Verification items for the finished model (mm, model axes). Face numbers are marked on the shaded views. A direction names the side the tool comes from. Coordinates: 2 decimals unless noted, no trailing zeros. Order: outer loops, then holes, each group sorted by start corner. A loop starts at its lowest first (then second) coordinate and runs counter-clockwise, first axis right, second up. Notation, with made-up numbers: M 25,5 L 70,5 A7 cw 70,16 Z; hole C 70.25,-39 d7. An arc over 180 degrees is marked long. Return JSON: item names as keys, results as strings. Group by question number.
Q1. Section check A-A, the plane y = 0. Enter the section's corners in (x, z).
Q2. Thickness scan on probe 1 along X at (y, z) = (-0.3, -0.25); probe 2 along Y at (x, z) = (3.25, -2.25); probe 3 along Y at (x, z) = (-3.5, -1.5). Record the ranges inside material, lowest first.
Q3. Go/stop test with flat-tipped pins: pin 1 Ø2 at (x, z) = (-3.5, -2) entering from -Y; pin 2 Ø3 at (x, z) = (1.5, 2) entering from -Y; pin 3 Ø1.5 at (x, y) = (-0.5, 1) entering from -Z. Record where each tip stops, or that it passes through.
Q4. Mould release check, pull along Y, two halves, no side actions. Record for the marked faces 3, 4 and 5: pulls with the +Y half, pulls with the -Y half, needs draft (parallel to the pull), parting line crosses it, or undercut.
Q5. Section check B-B, the plane x = 2.25. Enter the section's corners in (y, z).
Q6. Section check C-C, the plane x = 0.5. Enter the section's corners in (y, z), then the cut area to 3 significant figures.
Q7. Access from +Z, -Z, +X, -X, +Y, -Y to the whole of each face (thin tool, end or side, straight path). Record for the marked faces 1 and 2.
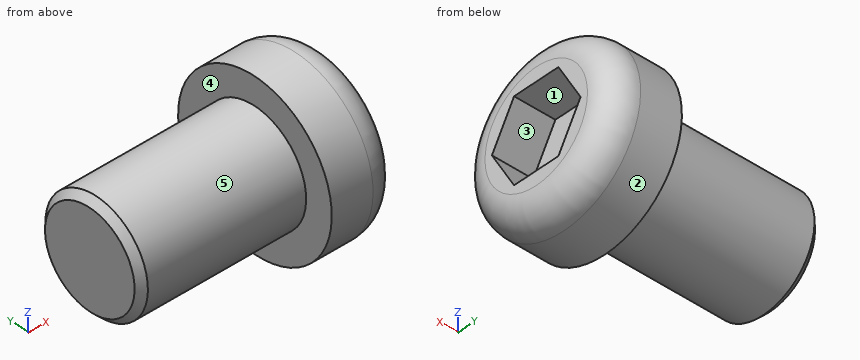
from build123d import *

# Parameters (mm, degrees)
F2_SIZE2 = 0.25
F2_SIZE  = 0.25
F3_R     = 1
F5_DEPTH = 1.5


with BuildPart() as f1:
    # F0 (on Front) → F1 (revolve)
    with BuildSketch(Plane.XZ):
        Polygon((4.25, 0), (-4.25, 0), (-4.25, -2), (1.75, -2), (1.75, -3), (4.25, -3), align=None)
    revolve(axis=Axis((4.160319, 0, 0), (1, 0, 0)))

    # F2
    f2_edges = [f1.edges().sort_by_distance(p)[0] for p in [
        (-4.25, 0, 2),
    ]]
    chamfer(f2_edges, length=F2_SIZE, length2=F2_SIZE2)

    # F3
    f3_edges = [f1.edges().sort_by_distance(p)[0] for p in [
        (4.25, 0, 3),
    ]]
    fillet(f3_edges, radius=F3_R)

    # F4 (on face) → F5 (cut)
    with BuildSketch(Plane.YZ.offset(4.25)):
        Polygon((0.866025, 1.5), (-0.866025, 1.5), (-1.732051, 0), (-0.866025, -1.5), (0.866025, -1.5), (1.732051, 0), align=None)
    extrude(amount=-F5_DEPTH, mode=Mode.SUBTRACT)


solid = f1.part
Numbers:
{
 "1": {"outline": "M -4.25,-1.75 L -4,-2 L 1.75,-2 L 1.75,-3 L 3.25,-3 A1 ccw 4.25,-2 L 4.25,-1.5 L 2.75,-1.5 L 2.75,1.5 L 4.25,1.5 L 4.25,2 A1 ccw 3.25,3 L 1.75,3 L 1.75,2 L -4,2 L -4.25,1.75 Z"},
 "2": {"probe 1": "x = -4.25 to 2.75", "probe 2": "y = -1.98 to 1.98", "probe 3": "y = -1.32 to 1.32"},
 "3": {"pin 1": "stops at y = -1.73", "pin 2": "stops at y = -2.95", "pin 3": "stops at z = -1.98"},
 "4": {"face 3": "undercut", "face 4": "needs draft", "face 5": "parting line crosses it"},
 "5": {"outline": "C 0,0 d6"},
 "6": {"outline": "C 0,0 d4", "area": "12.6 mm2"},
 "7": {"face 1": "+X", "face 2": "+X, -X"}
}
